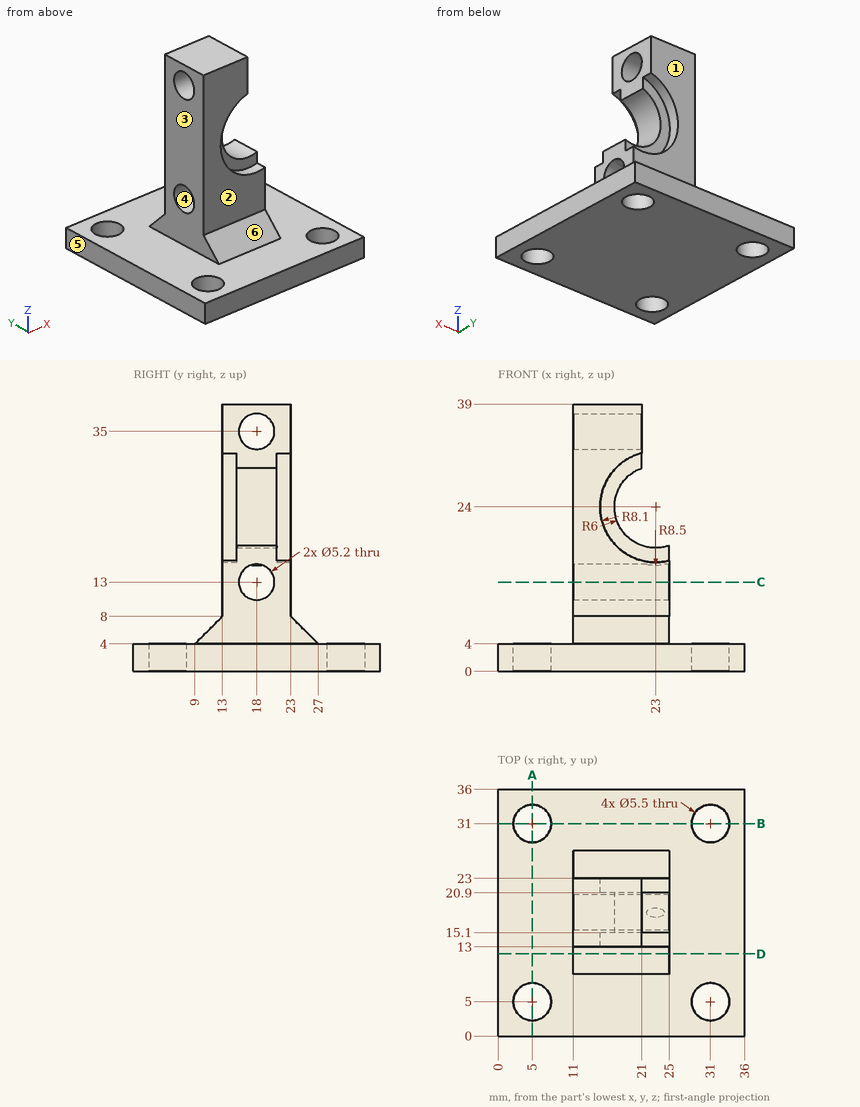
Drawing for the job (mm, zero at the part's lowest x, y, z). A direction names the side the tool comes from. Round coordinates to 2 decimals unless told otherwise and drop trailing zeros. Order: outer loops, then holes, each group sorted by start corner. A loop starts at its lowest first (then second) coordinate and runs counter-clockwise, first axis right, second up. Notation, with made-up numbers: (82.5, 43.25) -> (115.5, 43.25) arc R16 ccw to (115.5, 73.25) -> close; hole circle Ø11 at (-27, 81). An arc over 180 degrees is marked (long way). Write item = value, one per line. Start each with the question number.
(1) Cut at D-D, the plane y = 12. List the corners of the cut face in (x, z), then the cut area to 3 significant figures.
(2) Pin check, flat tips, straight feed: P1, Ø7, axis at x = 19, z = 28, coming from the +Y side; P2, Ø9, axis at y = 18.5, z = 25.5, coming from the -X side; P3, Ø8, axis at x = 20.5, z = 21, coming from the +Y side. Stop position of each tip, or through.
(3) Which spindle directions (+Z, -Z, +X, -X, +Y, -Y) get a long thin tool onto all of the face, cutting with end or side? Do the marked faces 1, 2 and 3. Say none if no direction does.
(4) Cut at A-A, the plane x = 5. List the corners of the cut face in (y, z), then the cut area to 3 significant figures.
(5) Pull direction Y, two halves, no side cores. Call the marked faces 4, 5 and 6: released by +Y, released by -Y, zero draft, split by the parting line, or undercut.
(6) Cut at C-C, the plane z = 13. List the corners of the cut face in (x, y), then the cut area to 3 significant figures.
(7) Probe line 1 (Y direction, x = 31, z = 2.95); line 2 (Y direction, x = 17, z = 35). List the from-to ranges inside material, lowest first. Write a range as [from, to].
Model answer:
q1.outline = (0, 0) -> (36, 0) -> (36, 4) -> (25, 4) -> (25, 7) -> (11, 7) -> (11, 4) -> (0, 4) -> close
q1.area = 186 mm2
q2.P1 = 23
q2.P2 = 11
q2.P3 = 20.9
q3.face_1 = +Z, +X, -X, +Y
q3.face_2 = +Z, +X, -X, -Y
q3.face_3 = +Z, -X, +Y, -Y
q4.outline = (0, 0) -> (2.25, 0) -> (2.25, 4) -> (0, 4) -> close; (7.75, 0) -> (28.25, 0) -> (28.25, 4) -> (7.75, 4) -> close; (33.75, 0) -> (36, 0) -> (36, 4) -> (33.75, 4) -> close
q4.area = 100 mm2
q5.face_4 = undercut
q5.face_5 = zero draft
q5.face_6 = released by -Y
q6.outline = (11, 13) -> (25, 13) -> (25, 15.4) -> (11, 15.4) -> close; (11, 20.6) -> (25, 20.6) -> (25, 23) -> (11, 23) -> close
q6.area = 67.2 mm2
q7.line_1 = [0, 2.25], [7.75, 28.25], [33.75, 36]
q7.line_2 = [13, 15.4], [20.6, 23]
